Check sheet for the modelled part. Datum: model origin and axes. Units: mm. Face numbers are marked on the shaded views. A direction names the side the tool comes from. Give positions to 0.01 mm unless a question says otherwise; leave off trailing zeros. Write each loop counter-clockwise with the first axis right and the second up, starting at its lowest first coordinate (ties: lowest second). Pieces come first, ordered by that corner, then holes. Notation, with made-up numbers: (31.25, -29) - (68.25, -29) arc R16 ccw to (68.25, -20) - close; hole circle Ø2 at (-35.5, 51.5). An arc over 180 degrees is marked (long way). Return JSON: item names as keys, results as strings. Group by question number.
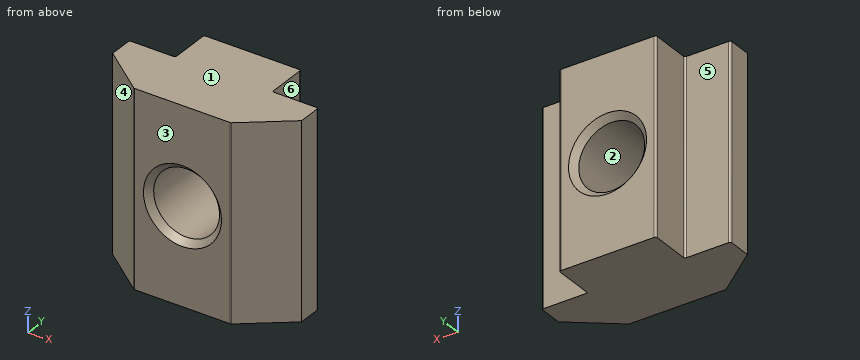
```python
from build123d import *

# Parameters (mm, degrees)
EXTRUDE_1_DEPTH = 10
FILLET_1_R      = 0.2


with BuildPart() as part:
    # Эскиз1 → Бобышка-Вытянуть1 (new body, symmetric)
    with BuildSketch(Plane.XY):
        Polygon((5, 0), (-5, 0), (-5, -4.3), (-9.75, -4.3), (-9.75, -6.8), (-5, -10.5), (5, -10.5), (9.75, -6.8), (9.75, -4.3), (5, -4.3), align=None)
    extrude(amount=EXTRUDE_1_DEPTH, both=True)

    # Эскиз4 → Отверстие обработанное метчиком M83 (revolve, cut)
    with BuildSketch(Plane(origin=(0, 0, 0), x_dir=(0, 0, 1), z_dir=(1, 0, 0))):
        Polygon((0, 0), (0, 10.5), (4.025, 10.5), (3.4, 9.875), (3.4, 0.625), (4.025, 0), align=None)
    revolve(axis=Axis((0, 6.35, 0), (0, -1, 0)), mode=Mode.SUBTRACT)

    # Скругление1
    fillet_1_edges = [part.edges().sort_by_distance(p)[0] for p in [
        (-5, 0, 0),
        (5, 0, 0),
        (5, -4.3, 0),
        (9.75, -4.3, 0),
        (5, -10.5, 0),
        (-5, -10.5, 0),
        (-9.75, -4.3, 0),
        (-5, -4.3, 0),
    ]]
    fillet(fillet_1_edges, radius=FILLET_1_R)


solid = part.part
```
Item 1: Section check D-D on z = 5.5. Record the cut outline in (x, y), plus the area to 3 significant figures.
Item 2: Material ranges on line 1 along X through (y, z) = (-4.5, 0); line 2 along Z through (x, y) = (0, -7.5), recorded low to high. Write a range as from..to.
Item 3: Depth check by flat-ended pin: pin 1 (3.5 mm diameter, centred on x = -8, z = -4, fed in from +Y); pin 2 (1.9 mm diameter, centred on y = -1, z = -1, fed in from +X); pin 3 (4.5 mm diameter, centred on y = -1.5, z = 3, fed in from -X). Enter the tip coordinate at first touch or a pass-through.
Item 4: Section check C-C on y = -3.25. Record the cut outline in (x, z).
Item 5: Section check A-A on x = 0. Record the cut outline in (y, z) (3 decimals), plus the area to 3 significant figures.
Item 6: Access from +Z, -Z, +X, -X, +Y, -Y to the whole of each face (thin tool, end or side, straight path). Record for the marked faces 4, 5 and 6.
Item 7: Section check B-B on z = 0. Record the cut outline in (x, y) (3 decimals).
Item 8: Mould release check, pull along Z, two halves, no side actions. Record for the marked faces 1, 2 and 3: +Z half, -Z half, draft (parallel to the pull), parting line (faces both ways), or undercut.
Reply:
{
 "1": {"outline": "(-9.75, -6.8) - (-5.05, -10.46) arc R0.2 ccw to (-4.93, -10.5) - (4.93, -10.5) arc R0.2 ccw to (5.05, -10.46) - (9.75, -6.8) - (9.75, -4.5) arc R0.2 ccw to (9.55, -4.3) - (5.2, -4.3) arc R0.2 cw to (5, -4.1) - (5, -0.2) arc R0.2 ccw to (4.8, 0) - (-4.8, 0) arc R0.2 ccw to (-5, -0.2) - (-5, -4.1) arc R0.2 cw to (-5.2, -4.3) - (-9.55, -4.3) arc R0.2 ccw to (-9.75, -4.5) - close", "area": "146 mm²"},
 "2": {"line 1": "-9.75..-3.4, 3.4..9.75", "line 2": "-10..-3.4, 3.4..10"},
 "3": {"pin 1": "y = -4.3", "pin 2": "x = 5", "pin 3": "x = -5"},
 "4": {"outline": "(-5, -10) - (5, -10) - (5, 10) - (-5, 10) - close; hole circle Ø6.8 at (0, 0)"},
 "5": {"outline": "(-10.5, -10) - (0, -10) - (0, -4.025) - (-0.625, -3.4) - (-9.875, -3.4) - (-10.5, -4.025) - close; (-10.5, 4.025) - (-9.875, 3.4) - (-0.625, 3.4) - (0, 4.025) - (0, 10) - (-10.5, 10) - close", "area": "138 mm²"},
 "6": {"face 4": "+Z, -Z, -X, -Y", "face 5": "+Z, -Z, -X, +Y", "face 6": "+Z, -Z, +X, +Y"},
 "7": {"outline": "(-9.75, -6.8) - (-5.054, -10.458) arc R0.2 ccw to (-4.931, -10.5) - (-4.025, -10.5) - (-3.4, -9.875) - (-3.4, -0.625) - (-4.025, 0) - (-4.8, 0) arc R0.2 ccw to (-5, -0.2) - (-5, -4.1) arc R0.2 cw to (-5.2, -4.3) - (-9.55, -4.3) arc R0.2 ccw to (-9.75, -4.5) - close; (3.4, -9.875) - (4.025, -10.5) - (4.931, -10.5) arc R0.2 ccw to (5.054, -10.458) - (9.75, -6.8) - (9.75, -4.5) arc R0.2 ccw to (9.55, -4.3) - (5.2, -4.3) arc R0.2 cw to (5, -4.1) - (5, -0.2) arc R0.2 ccw to (4.8, 0) - (4.025, 0) - (3.4, -0.625) - close"},
 "8": {"face 1": "+Z half", "face 2": "undercut", "face 3": "draft"}
}
